from build123d import *

# Parameters (mm, degrees)
EXTRUDE_1_DEPTH       = 2
CUT_EXTRUDE_1_DEPTH   = 1
CUT_EXTRUDE_2_DEPTH   = 1
CUT_EXTRUDE_3_DEPTH   = 1
CUT_EXTRUDE_4_DEPTH   = 1
HOLE_WIZARD_3_0_3_1_D = 3
HOLE_WIZARD_M421_D    = 46
FILLET_1_R            = 42


with BuildPart() as part:
    # Эскиз1 → Бобышка-Вытянуть1 (new body)
    with BuildSketch(Plane.XY.offset(-2)):
        Polygon((41.5, 6), (35.95120701, 35.95120701), (6, 41.5), (-6, 41.5), (-35.95120701, 35.95120701), (-41.5, 6), (-41.5, -6), (-35.95120701, -35.95120701), (-6, -41.5), (6, -41.5), (35.95120701, -35.95120701), (41.5, -6), align=None)
    extrude(amount=-EXTRUDE_1_DEPTH)

    # Эскиз2 → Вырез-Вытянуть1 (cut)
    with BuildSketch(Plane.XY.offset(-2)):
        with BuildLine():
            Line((9.5, -39.632688529), (10.5, -39.632688529))
            ThreePointArc((10.5, -39.632688529), (28.991378029, -28.991378029), (39.632688529, -10.5))
            Line((39.632688529, -10.5), (39.632688529, -9.5))
            Line((39.632688529, -9.5), (38.855501541, -9.5))
            ThreePointArc((38.855501541, -9.5), (28.284271247, -28.284271247), (9.5, -38.855501541))
            Line((9.5, -38.855501541), (9.5, -39.632688529))
        make_face()
    extrude(amount=-CUT_EXTRUDE_1_DEPTH, mode=Mode.SUBTRACT)

    # Эскиз3 → Вырез-Вытянуть2 (cut)
    with BuildSketch(Plane.XY.offset(-2)):
        with BuildLine():
            Line((-39.632688529, -9.5), (-39.632688529, -10.5))
            ThreePointArc((-39.632688529, -10.5), (-28.991378029, -28.991378029), (-10.5, -39.632688529))
            Line((-10.5, -39.632688529), (-9.5, -39.632688529))
            Line((-9.5, -39.632688529), (-9.5, -38.855501541))
            ThreePointArc((-9.5, -38.855501541), (-28.284271247, -28.284271247), (-38.855501541, -9.5))
            Line((-38.855501541, -9.5), (-39.632688529, -9.5))
        make_face()
    extrude(amount=-CUT_EXTRUDE_2_DEPTH, mode=Mode.SUBTRACT)

    # Эскиз4 → Вырез-Вытянуть3 (cut)
    with BuildSketch(Plane.XY.offset(-2)):
        with BuildLine():
            Line((39.632688529, 9.5), (39.632688529, 10.5))
            ThreePointArc((39.632688529, 10.5), (28.991378029, 28.991378029), (10.5, 39.632688529))
            Line((10.5, 39.632688529), (9.5, 39.632688529))
            Line((9.5, 39.632688529), (9.5, 38.855501541))
            ThreePointArc((9.5, 38.855501541), (28.284271247, 28.284271247), (38.855501541, 9.5))
            Line((38.855501541, 9.5), (39.632688529, 9.5))
        make_face()
    extrude(amount=-CUT_EXTRUDE_3_DEPTH, mode=Mode.SUBTRACT)

    # Эскиз5 → Вырез-Вытянуть4 (cut)
    with BuildSketch(Plane.XY.offset(-2)):
        with BuildLine():
            Line((-9.5, 39.632688529), (-10.5, 39.632688529))
            ThreePointArc((-10.5, 39.632688529), (-28.991378029, 28.991378029), (-39.632688529, 10.5))
            Line((-39.632688529, 10.5), (-39.632688529, 9.5))
            Line((-39.632688529, 9.5), (-38.855501541, 9.5))
            ThreePointArc((-38.855501541, 9.5), (-28.284271247, 28.284271247), (-9.5, 38.855501541))
            Line((-9.5, 38.855501541), (-9.5, 39.632688529))
        make_face()
    extrude(amount=-CUT_EXTRUDE_4_DEPTH, mode=Mode.SUBTRACT)

    # Диаметр отверстия Ø3.0 (3)1 (through all)
    with Locations(Plane.XY.offset(-2)):
        with Locations((32.291639785, -13.5), (32.291639785, 13.5), (19.798989873, 19.798989873), (19.798989873, -19.798989873), (13.5, -32.291639785), (-13.5, -32.291639785), (-19.798989873, -19.798989873), (-19.798989873, 19.798989873), (-13.5, 32.291639785), (13.5, 32.291639785), (-32.291639785, 13.5), (-32.291639785, -13.5)):
            Hole(HOLE_WIZARD_3_0_3_1_D / 2)

    # Отверстие с зазором M421 (through all)
    with Locations(Plane.XY.offset(-2)):
        with Locations((0, 0)):
            Hole(HOLE_WIZARD_M421_D / 2)

    # Скругление1
    fillet_1_edges = [part.edges().sort_by_distance(p)[0] for p in [
        (35.95120701, -35.95120701, -3),
        (-35.95120701, -35.95120701, -3),
        (-35.95120701, 35.95120701, -3),
        (35.95120701, 35.95120701, -3),
    ]]
    fillet(fillet_1_edges, radius=FILLET_1_R)


solid = part.part
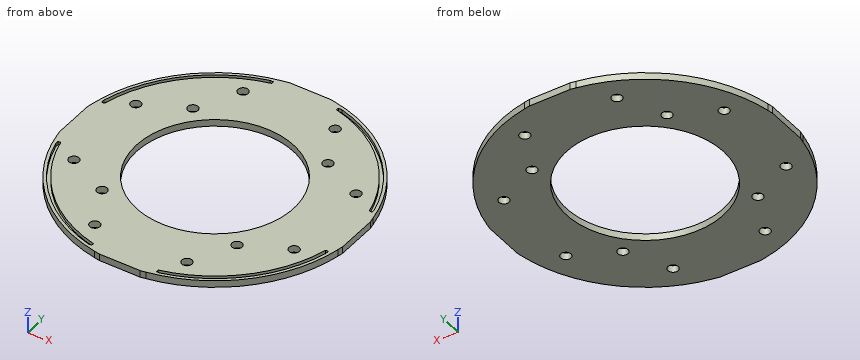
Geometry check sheet. Reference: the model listing, model coordinates, mm. Coordinates: 2 decimals unless noted, no trailing zeros. Write each loop counter-clockwise with the first axis right and the second up, starting at its lowest first coordinate (ties: lowest second). Pieces come first, ordered by that corner, then holes. Notation, with made-up numbers: (57.5, -16.75) -> (68.5, -16.75) arc R30 cw to (68.5, 21.25) -> close; hole circle Ø11 at (81, 11). An arc over 180 degrees is marked (long way). One line per question, with ' | ' between items.
1. Depth check by flat-ended pin: pin 1 Ø24 at (x, y) = (30.5, -27) entering from +Z; pin 2 Ø0.6 at (y, z) = (-39, -2.5) entering from -X; pin 3 Ø0.5 at (y, z) = (-10, -2.5) entering from -X; pin 4 Ø1 at (y, z) = (-24, -2.5) entering from +X. Enter the tip coordinate at first touch or a pass-through.
Answers:
pin 1: stops at z = -2 | pin 2: stops at x = -16.02 | pin 3: stops at x = -40.74 | pin 4: stops at x = 34.66
2. Cross-section at D-D on x = 20. Record the cut outline in (y, z), and give its area (3 significant figures).
Answers:
outline: (-36.8, -4) -> (-21.29, -4) -> (-21.29, -2) -> (-34.64, -2) -> (-34.64, -3) -> (-35.79, -3) -> (-35.79, -2) -> (-36.8, -2) -> close; (-18.31, -4) -> (-11.36, -4) -> (-11.36, -2) -> (-18.31, -2) -> close; (11.36, -4) -> (18.31, -4) -> (18.31, -2) -> (11.36, -2) -> close; (21.29, -4) -> (36.8, -4) -> (36.8, -2) -> (35.79, -2) -> (35.79, -3) -> (34.64, -3) -> (34.64, -2) -> (21.29, -2) -> close | area: 87.6 mm²
3. Thickness scan on probe 1 along X at (y, z) = (19, -2.9); probe 2 along X at (y, z) = (-18.5, -2.45); probe 3 along X at (y, z) = (14.5, -3.1). Record the ranges inside material, lowest first. Write a range as from..to.
Answers:
probe 1: x = -37.33..-36.33, -35.2..-21.07, -18.53..-12.96, 12.96..18.53, 21.07..35.2, 36.33..37.33 | probe 2: x = -37.58..-36.59, -35.46..-20.55, -19.05..-13.67, 13.67..19.05, 20.55..35.46, 36.59..37.58 | probe 3: x = -39.3..-33.41, -31.17..-17.85, 17.85..31.17, 33.41..39.3
4. Cross-section at C-C on y = 5. Record the cut outline in (x, z), and give its area (3 significant figures).
Answers:
outline: (-41.5, -4) -> (-22.45, -4) -> (-22.45, -2) -> (-41.5, -2) -> close; (22.45, -4) -> (41.5, -4) -> (41.5, -2) -> (22.45, -2) -> close | area: 76.2 mm²
5. Cross-section at B-B on y = 13.5. Record the cut outline in (x, z), and give its area (3 significant figures).
Answers:
outline: (-39.65, -4) -> (-33.79, -4) -> (-33.79, -2) -> (-37.65, -2) -> (-37.65, -3) -> (-38.71, -3) -> (-38.71, -2) -> (-39.65, -2) -> close; (-30.79, -4) -> (-18.62, -4) -> (-18.62, -2) -> (-30.79, -2) -> close; (18.62, -4) -> (30.79, -4) -> (30.79, -2) -> (18.62, -2) -> close; (33.79, -4) -> (39.65, -4) -> (39.65, -2) -> (38.71, -2) -> (38.71, -3) -> (37.65, -3) -> (37.65, -2) -> (33.79, -2) -> close | area: 70.0 mm²
6. Cross-section at A-A on x = 0. Record the cut outline in (y, z).
Answers:
outline: (-41.5, -4) -> (-23, -4) -> (-23, -2) -> (-41.5, -2) -> close; (23, -4) -> (41.5, -4) -> (41.5, -2) -> (23, -2) -> close
